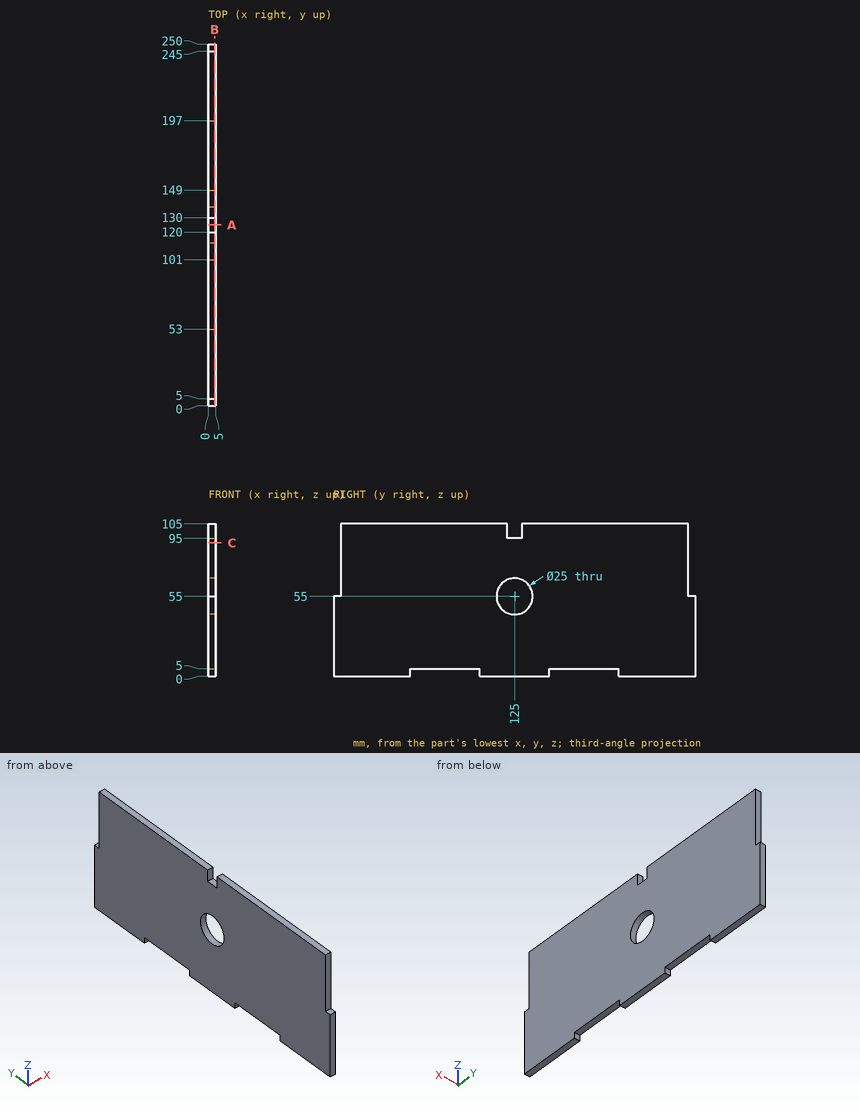
The drawing under review shows one solid part. Ordinate dimensions are in mm from its lowest x, y, z. Coordinates: 2 decimals unless noted, no trailing zeros. Write each loop counter-clockwise with the first axis right and the second up, starting at its lowest first coordinate (ties: lowest second). Pieces come first, ordered by that corner, then holes.
1) Insertion check: pin 1 (2.5 mm diameter, centred on x = 3, z = 79, fed in from +Y); pin 2 (2.5 mm diameter, centred on x = 3, y = 165, fed in from -Z); pin 3 (22.5 mm diameter, centred on y = 125, z = 55, fed in from -X); pin 4 (1.5 mm diameter, centred on x = 2.5, y = 248.5, fed in from +Z). Each pin has a flat end and moves straight along its axis. Give the tip position at first contact, or say it passes through.
2) Add section B-B (x = 4.25). Write out the cut boundary in (y, z), plus the area to 3 significant figures.
3) Add section A-A (y = 125). Write out the cut boundary in (x, z).
4) Add section C-C (z = 92). Write out the cut boundary in (x, y).
5) To check wall thickness, follow L1, parallel to Z at x = 2.7, y = 125; L2, parallel to Y at x = 2, z = 49; L3, parallel to Y at x = 3.15, z = 97. State the ranges of each line that lie inside material, in increasing order.
Check result:
1. pin 1: stops at y = 245
1. pin 2: stops at z = 5
1. pin 3: passes through
1. pin 4: stops at z = 55
2. outline: (0, 0) - (53, 0) - (53, 5) - (101, 5) - (101, 0) - (149, 0) - (149, 5) - (197, 5) - (197, 0) - (250, 0) - (250, 55) - (245, 55) - (245, 105) - (130, 105) - (130, 95) - (120, 95) - (120, 105) - (5, 105) - (5, 55) - (0, 55) - close; hole circle Ø25 at (125, 55)
2. area: 24,700 mm2
3. outline: (0, 0) - (5, 0) - (5, 42.5) - (0, 42.5) - close; (0, 67.5) - (5, 67.5) - (5, 95) - (0, 95) - close
4. outline: (0, 5) - (5, 5) - (5, 245) - (0, 245) - close
5. L1: z = 0 to 42.5, 67.5 to 95
5. L2: y = 0 to 114.03, 135.97 to 250
5. L3: y = 5 to 120, 130 to 245
